Verification items for the finished model (mm, model axes). Round coordinates to 2 decimals unless told otherwise and drop trailing zeros. Order: outer loops, then holes, each group sorted by start corner. A loop starts at its lowest first (then second) coordinate and runs counter-clockwise, first axis right, second up.
```python
from build123d import *

# Parameters (mm, degrees)
F1_DEPTH = 6.35
F2_DEPTH = 39.497
F3_SIZE2 = 4.2672
F3_SIZE  = 2.7178
F4_R     = 5.08


# Not quite as in the source:
# - a fillet or chamfer that OpenCascade refuses, or shapes differently, is made with other operations: its cross-section is extruded or revolved along the edge and cut away or added


with BuildPart() as f1:
    # F0 (on Right) → F1 (new body)
    with BuildSketch(Plane.YZ):
        with BuildLine():
            Line((0, 79.375), (-25.4, 79.375))
            Line((-25.4, 79.375), (-25.4, -79.375))
            Line((-25.4, -79.375), (0, -79.375))
            Line((0, -79.375), (0, -68.7324))
            ThreePointArc((0, -68.7324), (-2.0574, -66.675), (0, -64.6176))
            Line((0, -64.6176), (0, -53.975))
            Line((0, -53.975), (0, -41.275))
            Line((0, -41.275), (0, 15.875))
            ThreePointArc((0, 15.875), (-12.7, 28.575), (0, 41.275))
            Line((0, 41.275), (0, 79.375))
        make_face()
        with BuildLine():
            Line((25.4, 79.375), (0, 79.375))
            Line((0, 79.375), (0, 41.275))
            ThreePointArc((0, 41.275), (8.9802561211, 37.5552561211), (12.7, 28.575))
            ThreePointArc((12.7, 28.575), (8.9802561211, 19.5947438789), (0, 15.875))
            Line((0, 15.875), (0, -41.275))
            Line((0, -41.275), (0, -53.975))
            Line((0, -53.975), (0, -64.6176))
            ThreePointArc((0, -64.6176), (1.4548014916, -65.2201985084), (2.0574, -66.675))
            ThreePointArc((2.0574, -66.675), (1.4548014916, -68.1298014916), (0, -68.7324))
            Line((0, -68.7324), (0, -79.375))
            Line((0, -79.375), (25.4, -79.375))
            Line((25.4, -79.375), (25.4, 79.375))
        make_face()
        with BuildLine():
            Line((0, 34.925), (0, 41.275))
            ThreePointArc((0, 41.275), (-12.7, 28.575), (0, 15.875))
            Line((0, 15.875), (0, 22.225))
            ThreePointArc((0, 22.225), (-6.35, 28.575), (0, 34.925))
        make_face()
        with BuildLine():
            ThreePointArc((12.7, 28.575), (8.9802561211, 37.5552561211), (0, 41.275))
            Line((0, 41.275), (0, 34.925))
            ThreePointArc((0, 34.925), (4.4901280605, 33.0651280605), (6.35, 28.575))
            ThreePointArc((6.35, 28.575), (4.4901280605, 24.0848719395), (0, 22.225))
            Line((0, 22.225), (0, 15.875))
            ThreePointArc((0, 15.875), (8.9802561211, 19.5947438789), (12.7, 28.575))
        make_face()
    extrude(amount=F1_DEPTH)

    # F0 (on Right) → F2 (join)
    with BuildSketch(Plane.YZ):
        with BuildLine():
            Line((0, 34.925), (0, 41.275))
            ThreePointArc((0, 41.275), (-12.7, 28.575), (0, 15.875))
            Line((0, 15.875), (0, 22.225))
            ThreePointArc((0, 22.225), (-6.35, 28.575), (0, 34.925))
        make_face()
        with BuildLine():
            ThreePointArc((12.7, 28.575), (8.9802561211, 37.5552561211), (0, 41.275))
            Line((0, 41.275), (0, 34.925))
            ThreePointArc((0, 34.925), (4.4901280605, 33.0651280605), (6.35, 28.575))
            ThreePointArc((6.35, 28.575), (4.4901280605, 24.0848719395), (0, 22.225))
            Line((0, 22.225), (0, 15.875))
            ThreePointArc((0, 15.875), (8.9802561211, 19.5947438789), (12.7, 28.575))
        make_face()
    extrude(amount=F2_DEPTH)

    # F3
    f3_edges = [f1.edges().sort_by_distance(p)[0] for p in [
        (0, 0, -68.7324),
    ]]
    f3_side = f1.faces().sort_by_distance((0, 0, -0.344897))[0]
    chamfer(f3_edges, length=F3_SIZE, length2=F3_SIZE2, reference=f3_side)

    # F4
    f4_edges = [f1.edges().sort_by_distance(p)[0] for p in [
        (6.35, 0, 41.275),
    ]]
    fillet(f4_edges, radius=F4_R)

    # F5: fillet of radius 2.54 on 1 edges, made by hand

    # F5_s1 → F5_t2 (revolve, cut)
    with BuildSketch(Plane.XZ):
        with BuildLine():
            ThreePointArc((39.497, 37.465), (38.7530512242, 35.6689487758), (36.957, 34.925))
            Line((36.957, 34.925), (39.497, 34.925))
            Line((39.497, 34.925), (39.497, 37.465))
        make_face()
    revolve(axis=Axis((39.497, 0, 28.575), (-1, 0, 0)), mode=Mode.SUBTRACT)


solid = f1.part
```
1) Draft check along Y on faces 1 (the flat face through (3, -25.4, 1)), 2 (the flat face through (39.497, -9, 26)), 3 (the cylindrical face through (18.22, 0.28, 22.23)). Enter one of: released by +Y, released by -Y, zero draft, split by the parting line, or undercut.
2) Sectioned sample at A-A on x = 26. Record the cut outline in (y, z) (3 decimals).
3) Sectioned sample at B-B on z = 3.5. Record the cut outline in (x, y), then the cut area to 3 significant figures.
4) Go/stop test with flat-tipped pins: pin 1 Ø10 at (x, z) = (21.5, 28.5) entering from +Y; pin 2 Ø1.5 at (y, z) = (6, 32.5) entering from +X; pin 3 Ø10 at (x, z) = (27.5, 41) entering from +Y. Record where each tip stops, or that it passes through.
5) Scan lines: probe 1 along Z at (x, y) = (37, 0) (3 decimals); probe 2 along X at (y, z) = (1, 48); probe 3 along Y at (x, z) = (12.5, 23.5). Record each from-to range of solid material in increasing order.
Returned:
1. face 1: released by -Y
1. face 2: zero draft
1. face 3: undercut
2. outline: circle Ø25.4 at (0, 28.575); hole circle Ø12.7 at (0, 28.575)
3. outline: (0, -25.4) - (6.35, -25.4) - (6.35, 25.4) - (0, 25.4) - close
3. area: 323 mm2
4. pin 1: stops at y = 12.7
4. pin 2: stops at x = 39.3
4. pin 3: stops at y = 10.3
5. probe 1: z = 15.875 to 22.225, 34.925 to 41.275
5. probe 2: x = 0 to 6.35
5. probe 3: y = -11.64 to -3.82, 3.82 to 11.64
